Design review of the part built by this model. Coordinates are the model's own, in mm. Face numbers are marked on the shaded views. A direction names the side the tool comes from. Give positions to 0.01 mm unless a question says otherwise; leave off trailing zeros. Write each loop counter-clockwise with the first axis right and the second up, starting at its lowest first coordinate (ties: lowest second). Pieces come first, ordered by that corner, then holes. Notation, with made-up numbers: (87, 0.5) - (97, 0.5) arc R23 cw to (97, 36.5) - close; hole circle Ø7 at (44.5, 6.25). An arc over 180 degrees is marked (long way). Write each question's results on one line, items separated by ' | '. Start each with the question number.
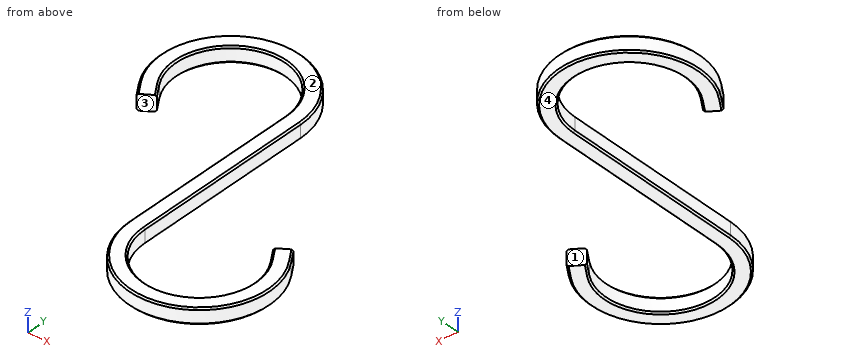
from build123d import *

# Parameters (mm, degrees)
F1_W    = 5
F1_H    = 5
F3_SIZE = 0.5


with BuildPart() as f2:
    # F2: sweep along a path in F0
    with BuildLine(Plane.XY) as f2_path:
        Line((-33.7847869337, 13.8033740678), (-36.5807514511, 17.9485619306))
        ThreePointArc((-36.5807514511, 17.9485619306), (-25.8474340945, 48.2585151193), (0, 29.13242))
        Line((0, 29.13242), (0, -29.13242))
        ThreePointArc((0, -29.13242), (25.8474340945, -48.2585151193), (36.5807514511, -17.9485619306))
        Line((36.5807514511, -17.9485619306), (33.7847869337, -13.8033740678))
    # F1 (on Front) → F2 (sweep)
    with BuildSketch(Plane.XZ):
        Rectangle(F1_W, F1_H)
    sweep(path=f2_path.line)

    # F3
    f3_edges = [f2.edges().sort_by_distance(p)[0] for p in [
        (-2.5, 0, -2.5),
        (-26.578363, 50.649277, -2.5),
        (-26.578363, 50.649277, 2.5),
        (-2.5, 0, 2.5),
    ]]
    chamfer(f3_edges, length=F3_SIZE)


solid = f2.part
Q1. The part is to be moulded in two halves that separate along X. For the marked faces 1 and 2, say which applies: +X half, -X half, draft (parallel to the pull), parting line (faces both ways), or undercut.
Q2. Add section B-B on x = -20. State the section outline as (y, z) points, plus the area to 3 significant figures.
Q3. Add section A-A on y = 9. State the section outline as (x, z) points.
Q4. For line 1 along X through (y, z) = (1, 1.1); line 2 along X through (y, z) = (-17.5, -0.4); line 3 along X through (y, z) = (43.5, -1.2), list the stretches that pass through material, from the lowest coordinate up. Write a range as [from, to].
Q5. Machinability: for the marked faces 3 and 4, which of the approach directions +Z, -Z, +X, -X, +Y, -Y give a long, thin tool a straight path to every point of the face, cutting with its end or side? Answer none if there is none.
Q6. Add section C-C on z = -1.05. State the section outline as (x, y) points.
Q7. Insertion check: P1, Ø1.5, axis at y = 14.5, z = 0, coming from the -X side; P2, Ø1.5, axis at x = -15, z = 1, coming from the -Y side; P3, Ø3, axis at x = -1, z = 2, coming from the -Y side. Each pin has a flat end and moves straight along its axis. Give the tip position at first contact, or say it passes through.
Result:
1) face 1: undercut | face 2: draft
2) outline: (46.63, -2) - (47.13, -2.5) - (51.13, -2.5) - (51.63, -2) - (51.63, 2) - (51.13, 2.5) - (47.13, 2.5) - (46.63, 2) - close | area: 24.5 mm²
3) outline: (-2.5, -2) - (-2, -2.5) - (2, -2.5) - (2.5, -2) - (2.5, 2) - (2, 2.5) - (-2, 2.5) - (-2.5, 2) - close
4) line 1: x = [-2.5, 2.5] | line 2: x = [-2.5, 2.5], [33.26, 39.26] | line 3: x = [-37.32, -29.99], [-10.01, -2.68]
5) face 3: +Z, -Z, -Y | face 4: -Z, +X, -X, +Y, -Y
6) outline: (-38.65, 16.55) - (-35.86, 12.41) - (-31.71, 15.2) - (-34.51, 19.35) arc R17.5 cw (long way) to (-2.5, 29.13) - (-2.5, -29.13) arc R22.5 ccw (long way) to (38.65, -16.55) - (35.86, -12.41) - (31.71, -15.2) - (34.51, -19.35) arc R17.5 cw (long way) to (2.5, -29.13) - (2.5, 29.13) arc R22.5 ccw (long way) to start
7) P1: stops at x = -37.78 | P2: stops at y = 45.66 | P3: stops at y = -40.36
